Can you work these out from the model? Positions are in its coordinate system, mm. A direction names the side the tool comes from. Coordinates: 2 decimals unless noted, no trailing zeros. Write each loop counter-clockwise with the first axis right and the second up, starting at its lowest first coordinate (ties: lowest second). Pieces come first, ordered by that corner, then holes. Notation, with made-up numbers: (74, 54) - (121, 54) arc R13 ccw to (121, 68) - close; hole circle Ø11 at (11.25, 84.25). An arc over 180 degrees is marked (long way). One line per question, with ' | ' between items. Start each with the question number.
from build123d import *

# Parameters (mm, degrees)
F0_W     = 22
F0_H     = 22
F1_DEPTH = 2
F2_R     = 1.55
F3_DEPTH = 2.001
F5_DEPTH = 12
F6_R     = 6.25
F6_R_2   = 4.25
F7_DEPTH = 12
F8_SIZE  = 1


with BuildPart() as f1:
    # F0 (on Top) → F1 (new body)
    with BuildSketch(Plane.XY):
        Rectangle(F0_W, F0_H)
    extrude(amount=F1_DEPTH)

    # F2 (on face) → F3 (cut, through all)
    with BuildSketch(Plane.XY.offset(2)):
        Circle(F2_R)
    extrude(amount=-F3_DEPTH, mode=Mode.SUBTRACT)

    # F4 (on face) → F5 (join)
    with BuildSketch(Plane(origin=(0, 0, 0), x_dir=(1, 0, 0), z_dir=(0, 0, -1))):
        Polygon((9, 11), (-9, 11), (-6, 8), (6, 8), align=None)
        Polygon((-8, 6), (-11, 9), (-11, -9), (-8, -6), align=None)
        Polygon((-6, -8), (-9, -11), (9, -11), (6, -8), align=None)
        Polygon((8, -6), (11, -9), (11, 9), (8, 6), align=None)
    extrude(amount=F5_DEPTH)

    # F6 (on face) → F7 (join)
    with BuildSketch(Plane.XZ.offset(11)):
        with Locations((0, -5)):
            Circle(F6_R)
        with Locations((0, -5)):
            Circle(F6_R_2, mode=Mode.SUBTRACT)
    extrude(amount=F7_DEPTH)

    # F8
    f8_edges = [f1.edges().sort_by_distance(p)[0] for p in [
        (-6.25, -23, -5),
    ]]
    chamfer(f8_edges, length=F8_SIZE)


solid = f1.part
(1) I'm going to push flat-ended pins straight in: pin 1 (4 mm diameter, centred on y = -11.5, z = -4, fed in from +X); pin 2 (3 mm diameter, centred on x = -6, z = -1.5, fed in from -Y); pin 3 (12 mm diameter, centred on x = 0.5, y = 4.5, fed in from -Z); pin 4 (4 mm diameter, centred on x = 0, y = 0, fed in from -Z). Where does each tip first touch, or does it pass through?
(2) If we section it at D-D on y = 5: List the corners of the cut face in (x, z) for me.
(3) If I drill on probe 1 along Z at (x, y) = (0, -19.5); probe 2 along Y at (x, z) = (-0.5, -4.5), over which ranges is the centre line in solid material (lowest first)?
(4) Which directions (+Z, -Z, +X, -X, +Y, -Y) give clear straight access to the entire face, cutting with the end or side of a thin tool? Please do faces 1 (the face through (0, -8, -6)), 2 (the face through (0, 9, -12)), 3 (the face through (-3, -11, 1)).
(5) If we section it at A-A on y = 0: List the corners of the cut face in (x, z) for me.
(6) If we section it at B-B on z = -5: List the corners of the cut face in (x, y) for me, plus the area to 3 significant figures.
(7) If we mould it in two halves opening along Z, with no side actions, what happens to faces 4 (the face through (0, -11, -5)), 5 (the face through (0, -10, -12)), 6 (the face through (10, -8, -6))? For each: +Z half, -Z half, draft (parallel to the pull), parting line (faces both ways), or undercut.
(8) If we section it at C-C on x = 0: List the corners of the cut face in (y, z) for me, plus the area to 3 significant figures.
Values:
1) pin 1: x = 9 | pin 2: y = -22.8 | pin 3: z = -12 | pin 4: z = 0
2) outline: (-11, -12) - (-8, -12) - (-8, 0) - (8, 0) - (8, -12) - (11, -12) - (11, 2) - (-11, 2) - close
3) probe 1: -11.25 to -9.25, -0.75 to 1.25 | probe 2: -11 to -8, 8 to 11
4) face 1: -Z | face 2: -Z, +X, -X, +Y, -Y | face 3: -Y
5) outline: (-11, -12) - (-8, -12) - (-8, 0) - (-1.55, 0) - (-1.55, 2) - (-11, 2) - close; (1.55, 0) - (8, 0) - (8, -12) - (11, -12) - (11, 2) - (1.55, 2) - close
6) outline: (-11, -9) - (-8, -6) - (-8, 6) - (-11, 9) - close; (-9, -11) - (-6.25, -11) - (-6.25, -22) - (-5.25, -23) - (-4.25, -23) - (-4.25, -11) - (4.25, -11) - (4.25, -23) - (5.25, -23) - (6.25, -22) - (6.25, -11) - (9, -11) - (6, -8) - (-6, -8) - close; (-9, 11) - (-6, 8) - (6, 8) - (9, 11) - close; (8, -6) - (11, -9) - (11, 9) - (8, 6) - close | area: 227 mm2
7) face 4: undercut | face 5: -Z half | face 6: draft
8) outline: (-23, -10.25) - (-22, -11.25) - (-11, -11.25) - (-11, -12) - (-8, -12) - (-8, 0) - (-1.55, 0) - (-1.55, 2) - (-11, 2) - (-11, 1.25) - (-22, 1.25) - (-23, 0.25) - (-23, -0.75) - (-11, -0.75) - (-11, -9.25) - (-23, -9.25) - close; (1.55, 0) - (8, 0) - (8, -12) - (11, -12) - (11, 2) - (1.55, 2) - close | area: 157 mm2
